Input: part model. Units: mm. Frame: model coordinates. A direction names the side the tool comes from. Coordinates: 2 decimals unless noted, no trailing zeros. Loops run counter-clockwise (first coordinate to the right, second up) from the corner with the lowest first, then second, coordinate; pieces in that order, holes last.
(1) Section D-D, the plane z = 22.5. Return loops of the section in (x, y).
(2) Section B-B, the plane y = 11.5. Return loops of the section in (x, z) (3 decimals), then the cut area to 3 significant figures.
(3) Set-up query: faces 4 (the face through (33.76, -0.36, 3.94)), 5 (the face through (5.401, 0, 13)), 6 (the face through (35, 0, -16)). Return all of +Z, -Z, +X, -X, +Y, -Y with unobstructed straight access to the full face (end or side cutting, diameter ignored); none if empty.
(4) Contact query for flat-ended pins moving along their axis: P1, Ø8, axis at y = 2.5, z = 19.5, coming from the -X side; P2, Ø6, axis at x = -20, z = -2, coming from the -Y side. Output: stop coordinate, or through.
(5) Section C-C, the plane z = -12.5. Return loops of the section in (x, y).
(6) Mould query, pull axis Y, two halves, no side actions, for faces 1 (the face through (35, -15.88, -16)), 2 (the face through (-20.35, -14.25, 1.18)), 3 (the face through (-45.399, 0, -4)). Classes: released by +Y, released by -Y, zero draft, split by the parting line, or undercut.
(7) Line query: L1, parallel to X at y = -5, z = -24.5; L2, parallel to X at y = -21, z = 25.5; L3, parallel to X at y = -4.5, z = 5. Output: solid intervals per line, ascending.
(8) Section A-A, the plane x = 37. Return loops of the section in (y, z), then the cut area to 3 significant figures.
```python
from build123d import *

# Parameters (mm, degrees)
F0_W     = 90.797476
F0_H     = 57.807724
F1_DEPTH = 25.4
F2_W     = 50.8
F2_H     = 57.807724
F2_R     = 14.940319
F3_DEPTH = 50.8
F5_D     = 6.35
F6_W     = 8.342021
F6_H     = 15.879793
F7_DEPTH = 25.4


with BuildPart() as f1:
    # F0 (on Front) → F1 (new body, symmetric)
    with BuildSketch(Plane.XZ):
        Rectangle(F0_W, F0_H)
    extrude(amount=F1_DEPTH, both=True)

    # F2 (on face) → F3 (cut)
    with BuildSketch(Plane(origin=(-45.398738, 0, 0), x_dir=(0, -1, 0), z_dir=(-1, 0, 0))):
        Rectangle(F2_W, F2_H)
        with Locations((0, -3.306166)):
            Circle(F2_R, mode=Mode.SUBTRACT)
    extrude(amount=-F3_DEPTH, mode=Mode.SUBTRACT)

    # F5 (through all)
    with Locations(Plane(origin=(0, 25.4, 0), x_dir=(-1, 0, 0), z_dir=(0, 1, 0))):
        with Locations((-30.731432, 2.991115)):
            Hole(F5_D / 2)

    # F6 (on face) → F7 (cut)
    with BuildSketch(Plane(origin=(0, 0, -28.903862), x_dir=(1, 0, 0), z_dir=(0, 0, -1))):
        with Locations((35.414792, 7.939896)):
            Rectangle(F6_W, F6_H)
    extrude(amount=-F7_DEPTH, mode=Mode.SUBTRACT)


solid = f1.part
```
Report:
1. outline: (5.4, -25.4) - (45.4, -25.4) - (45.4, 25.4) - (5.4, 25.4) - close
2. outline: (-45.399, -12.844) - (5.401, -12.844) - (5.401, -28.904) - (45.399, -28.904) - (45.399, 28.904) - (5.401, 28.904) - (5.401, 6.231) - (-45.399, 6.231) - close; hole circle Ø6.35 at (30.731, 2.991)
2. area: 3,250 mm2
3. face 4: +Y, -Y
3. face 5: -X
3. face 6: -Z
4. P1: stops at x = 5.4
4. P2: stops at y = -14.94
5. outline: (-45.4, -11.78) - (5.4, -11.78) - (5.4, -25.4) - (45.4, -25.4) - (45.4, 25.4) - (5.4, 25.4) - (5.4, 11.78) - (-45.4, 11.78) - close; hole (31.24, -15.88) - (39.59, -15.88) - (39.59, 0) - (31.24, 0) - close
6. face 1: undercut
6. face 2: split by the parting line
6. face 3: zero draft
7. L1: x = 5.4 to 31.24, 39.59 to 45.4
7. L2: x = 5.4 to 45.4
7. L3: x = -45.4 to 28.27, 33.19 to 45.4
8. outline: (-25.4, -28.9) - (-15.88, -28.9) - (-15.88, -3.5) - (0, -3.5) - (0, -28.9) - (25.4, -28.9) - (25.4, 28.9) - (-25.4, 28.9) - close
8. area: 2,530 mm2
